Can you work these out from the model? Positions are in its coordinate system, mm. A direction names the side the tool comes from. Coordinates: 2 decimals unless noted, no trailing zeros. Order: outer loops, then holes, each group sorted by start corner. A loop starts at its lowest first (then second) coordinate and runs counter-clockwise, first axis right, second up. Notation, with made-up numbers: (61, 63) - (115, 63) arc R15 cw to (115, 83) - close; hole circle Ø3 at (0.25, 56.5). An arc over 180 degrees is marked (long way). Use a Markdown table: item, result. Add a question column.
(1) We'd pull the mould along Y, two halves only. Please class faces 5 (the flat face through (8, 21.65, 27)), 6 (the cylindrical face through (13.45, 9.2, 6.27)), 7 (the cylindrical face through (9.262, 22.461, 27.196)): pulls with the +Y half, pulls with the -Y half, needs draft (parallel to the pull), parting line crosses it, or undercut.
(2) I want a section at D-D (z = 18.5). List the corners of the cut face in (x, y) for me.
(3) I want a section at A-A (z = 25). List the corners of the cut face in (x, y) for me.
(4) On a 3-axis mill with a long thin cutter (end or side, diameter ignored), from which of +Z, -Z, +X, -X, +Y, -Y can I reach the whole of each face in a straight line? I mean faces 1 (the flat face through (9, 17.25, 19)), 2 (the flat face through (3, 21.65, 19.2)), 3 (the cylindrical face through (13.64, 20.29, 29.1)), 4 (the flat face through (9, 6, 4.5)). Say none if no direction works.
(5) I want a section at C-C (y = 15.25). List the corners of the cut face in (x, z) for me.
(6) If I drill on L1, parallel to X at y = 19.25, z = 17.5; L2, parallel to Z at x = 9.75, y = 20.3; L3, parallel to Y at x = 7.25, z = 1.7, over which ranges is the centre line in solid material (lowest first)? Write a range as [from, to].
(7) I want a section at B-B (x = 10). List the corners of the cut face in (y, z) for me.
(8) For pin 1 Ø6 at (x, z) = (12, 19.5) entering from -Y; pin 2 Ø4 at (x, z) = (6, 16) entering from -Y; pin 3 Ø3.5 at (x, z) = (9.75, 25) entering from +Y; pin 4 Ø6.5 at (x, y) = (9.5, 5.5) entering from +Z, each with a flat end and sliding along its axis, tell me the tip position at first contact or that it passes through.
```python
from build123d import *

# Parameters (mm, degrees)
SKIZZE1_W                                            = 14.5
SKIZZE1_H                                            = 23.25
AUFSATZ_LINEAR_AUSTRAGEN1_DEPTH                      = 30
SKIZZE5_W                                            = 22
SKIZZE5_H                                            = 17.25
SCHNITT_LINEAR_AUSTRAGEN3_DEPTH                      = 41.630191976
VERRUNDUNG1_R                                        = 7.25
STIRNSENKUNG_F_R_M4_ZYLINDERSCHRAUBE_MIT_D           = 4.5
STIRNSENKUNG_F_R_M4_ZYLINDERSCHRAUBE_MIT_CBORE_D     = 8
STIRNSENKUNG_F_R_M4_ZYLINDERSCHRAUBE_MIT_CBORE_DEPTH = 4.4
SKIZZE9_R                                            = 6.5
SCHNITT_LINEAR_AUSTRAGEN4_DEPTH                      = 3.5
SKIZZE10_R                                           = 1.75
SCHNITT_LINEAR_AUSTRAGEN5_DEPTH                      = 5.5
SKIZZE11_OUTSIDE_W                                   = 24.626
SKIZZE11_OUTSIDE_H                                   = 40.126
SCHNITT_LINEAR_AUSTRAGEN6_DEPTH                      = 41.630191976


with BuildPart() as part:
    # Skizze1 → Aufsatz-Linear austragen1 (new body)
    with BuildSketch(Plane.XY):
        with Locations((7.25, 11.625)):
            Rectangle(SKIZZE1_W, SKIZZE1_H)
    extrude(amount=AUFSATZ_LINEAR_AUSTRAGEN1_DEPTH)

    # Skizze5 → Schnitt-Linear austragen3 (cut, through all)
    with BuildSketch(Plane(origin=(14.5, 0, 0), x_dir=(0, 0, -1), z_dir=(1, 0, 0))):
        with Locations((-19, 8.625)):
            Rectangle(SKIZZE5_W, SKIZZE5_H)
    extrude(amount=-SCHNITT_LINEAR_AUSTRAGEN3_DEPTH, mode=Mode.SUBTRACT)

    # Verrundung1
    verrundung1_edges = [part.edges().sort_by_distance(p)[0] for p in [
        (14.5, 0, 4),
        (0, 0, 4),
    ]]
    fillet(verrundung1_edges, radius=VERRUNDUNG1_R - 0.0001)  # a hair under: the kernel refuses the full size

    # Stirnsenkung für M4 Zylinderschraube mit Innensechskant1 (through all)
    with Locations(Plane(origin=(0, 17.25, 0), x_dir=(-1, 0, 0), z_dir=(0, -1, 0))):
        with Locations((-4.75, -17.5), (-9.75, -25)):
            CounterBoreHole(STIRNSENKUNG_F_R_M4_ZYLINDERSCHRAUBE_MIT_D / 2, STIRNSENKUNG_F_R_M4_ZYLINDERSCHRAUBE_MIT_CBORE_D / 2, STIRNSENKUNG_F_R_M4_ZYLINDERSCHRAUBE_MIT_CBORE_DEPTH)

    # Skizze9 → Schnitt-Linear austragen4 (cut)
    with BuildSketch(Plane.XY.offset(8)):
        with Locations((7.25, 7.25)):
            Circle(SKIZZE9_R)
    extrude(amount=-SCHNITT_LINEAR_AUSTRAGEN4_DEPTH, mode=Mode.SUBTRACT)

    # Skizze10 → Schnitt-Linear austragen5 (cut)
    with BuildSketch(Plane.XY.offset(4.5)):
        with Locations((7.25, 7.25)):
            Circle(SKIZZE10_R)
    extrude(amount=-SCHNITT_LINEAR_AUSTRAGEN5_DEPTH, mode=Mode.SUBTRACT)

    # Skizze11 outside → Schnitt-Linear austragen6 (cut, through all)
    with BuildSketch(Plane(origin=(0, 23.25, 0), x_dir=(1, 0, 0), z_dir=(0, 1, 0))):
        with Locations((7.25, -15)):
            Rectangle(SKIZZE11_OUTSIDE_W, SKIZZE11_OUTSIDE_H)
        with BuildLine():
            Line((3, 0), (11.5, 0))
            ThreePointArc((11.5, 0), (13.621320344, -0.878679656), (14.5, -3))
            Line((14.5, -3), (14.5, -27))
            ThreePointArc((14.5, -27), (13.621320344, -29.121320344), (11.5, -30))
            Line((11.5, -30), (3, -30))
            ThreePointArc((3, -30), (0.878679656, -29.121320344), (0, -27))
            Line((0, -27), (0, -3))
            ThreePointArc((0, -3), (0.878679656, -0.878679656), (3, 0))
        make_face(mode=Mode.SUBTRACT)
    extrude(amount=-SCHNITT_LINEAR_AUSTRAGEN6_DEPTH, mode=Mode.SUBTRACT)


solid = part.part
```
Answers follow:
| question | item | result |
|---|---|---|
| 1 | face 5 | pulls with the -Y half |
| 1 | face 6 | undercut |
| 1 | face 7 | needs draft |
| 2 | outline | (0, 17.25) - (0.88, 17.25) - (0.88, 21.65) - (2.73, 21.65) - (2.73, 23.25) - (0, 23.25) - close; (6.77, 21.65) - (8.62, 21.65) - (8.62, 17.25) - (14.5, 17.25) - (14.5, 23.25) - (6.77, 23.25) - close |
| 3 | outline | (0, 17.25) - (5.75, 17.25) - (5.75, 21.65) - (7.5, 21.65) - (7.5, 23.25) - (0, 23.25) - close; (12, 21.65) - (13.75, 21.65) - (13.75, 17.25) - (14.5, 17.25) - (14.5, 23.25) - (12, 23.25) - close |
| 4 | face 1 | +Z, +X, -X, -Y |
| 4 | face 2 | -Y |
| 4 | face 3 | +Z, +X, +Y, -Y |
| 4 | face 4 | +Z |
| 5 | outline | (0, 3) arc R3 ccw to (3, 0) - (11.5, 0) arc R3 ccw to (14.5, 3) - (14.5, 8) - (0, 8) - close |
| 6 | L1 | x = [0, 0.75], [8.75, 14.5] |
| 6 | L2 | z = [0, 21], [29, 30] |
| 6 | L3 | y = [0, 5.5], [9, 23.25] |
| 7 | outline | (0.54, 0) - (23.25, 0) - (23.25, 22.76) - (21.65, 22.76) - (21.65, 21.01) - (17.25, 21.01) - (17.25, 8) - (13.14, 8) - (13.14, 4.5) - (1.36, 4.5) - (1.36, 8) - (0.54, 8) - close; (17.25, 28.99) - (21.65, 28.99) - (21.65, 27.24) - (23.25, 27.24) - (23.25, 30) - (17.25, 30) - close |
| 8 | pin 1 | stops at y = 17.25 |
| 8 | pin 2 | stops at y = 21.65 |
| 8 | pin 3 | passes through |
| 8 | pin 4 | stops at z = 4.5 |
